```python
from build123d import *

# Parameters (mm, degrees)
SKETCH1_W           = 220
SKETCH1_H           = 145
BOSS_EXTRUDE1_DEPTH = 3
SKETCH2_W           = 220
SKETCH2_H           = 145
BOSS_EXTRUDE2_DEPTH = 12


with BuildPart() as part:
    # Sketch1 → Boss-Extrude1 (new body)
    with BuildSketch(Plane(origin=(0, 0, 0), x_dir=(1, 0, 0), z_dir=(0, 1, 0))):
        with Locations((110, 72.5)):
            Rectangle(SKETCH1_W, SKETCH1_H)
    extrude(amount=BOSS_EXTRUDE1_DEPTH)

    # Sketch2 → Boss-Extrude2 (add)
    with BuildSketch(Plane(origin=(0, 3, 0), x_dir=(1, 0, 0), z_dir=(0, 1, 0))):
        with Locations((110, 72.5)):
            Rectangle(SKETCH2_W, SKETCH2_H)
        with BuildLine():
            Line((3, 123.3), (3, 21.7))
            ThreePointArc((3, 21.7), (9.01040764, 19.21040764), (11.5, 13.2))
            Line((11.5, 13.2), (11.5, 3))
            Line((11.5, 3), (208.5, 3))
            Line((208.5, 3), (208.5, 13.2))
            ThreePointArc((208.5, 13.2), (210.98959236, 19.21040764), (217, 21.7))
            Line((217, 21.7), (217, 123.3))
            ThreePointArc((217, 123.3), (210.98959236, 125.78959236), (208.5, 131.8))
            Line((208.5, 131.8), (208.5, 142))
            Line((208.5, 142), (11.5, 142))
            Line((11.5, 142), (11.5, 131.8))
            ThreePointArc((11.5, 131.8), (9.01040764, 125.78959236), (3, 123.3))
        make_face(mode=Mode.SUBTRACT)
    extrude(amount=BOSS_EXTRUDE2_DEPTH)


solid = part.part
```
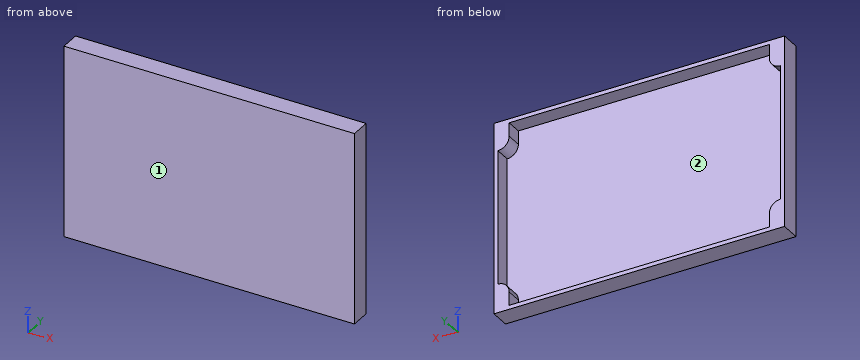
Check sheet for the modelled part. Datum: model origin and axes. Units: mm. Face numbers are marked on the shaded views. Give positions to 0.01 mm unless a question says otherwise; leave off trailing zeros. Write each loop counter-clockwise with the first axis right and the second up, starting at its lowest first coordinate (ties: lowest second). Pieces come first, ordered by that corner, then holes. Notation, with made-up numbers: (33.5, -15.5) - (91.5, -15.5) arc R29 ccw to (91.5, 9.5) - close; hole circle Ø2 at (67.5, 0). An arc over 180 degrees is marked (long way). Answer as a JSON object with one key per item and string values. Group by question number.
1) Sectioned sample at A-A (y = 6). Record the cut outline in (x, z).
2) Sectioned sample at B-B (z = -39). Record the cut outline in (x, y).
3) Release check for a two-part mould opening along Z. For the marked faces 1 and 2 record: pulls with the +Z half, pulls with the -Z half, needs draft (parallel to the pull), parting line crosses it, or undercut.
4) Depth check by flat-ended pin: P1, Ø1.5, axis at x = 47.5, z = -73.5, coming from the +Y side. Enter the tip coordinate at first touch or a pass-through.
5) Thickness scan on probe 1 along Z at (x, y) = (185.5, 5.25); probe 2 along X at (y, z) = (4, -46); probe 3 along X at (y, z) = (6.5, -136). Record the ranges inside material, lowest first. Write a range as from..to.
6) Sectioned sample at C-C (x = 169). Record the cut outline in (y, z), then the cut area to 3 significant figures.
Geometry results:
{
 "1": {"outline": "(0, -145) - (220, -145) - (220, 0) - (0, 0) - close; hole (3, -123.3) arc R8.5 cw to (11.5, -131.8) - (11.5, -142) - (208.5, -142) - (208.5, -131.8) arc R8.5 cw to (217, -123.3) - (217, -21.7) arc R8.5 cw to (208.5, -13.2) - (208.5, -3) - (11.5, -3) - (11.5, -13.2) arc R8.5 cw to (3, -21.7) - close"},
 "2": {"outline": "(0, 0) - (220, 0) - (220, 15) - (217, 15) - (217, 3) - (3, 3) - (3, 15) - (0, 15) - close"},
 "3": {"face 1": "needs draft", "face 2": "undercut"},
 "4": {"P1": "stops at y = 3"},
 "5": {"probe 1": "z = -145..-142, -3..0", "probe 2": "x = 0..3, 217..220", "probe 3": "x = 0..11.5, 208.5..220"},
 "6": {"outline": "(0, -145) - (15, -145) - (15, -142) - (3, -142) - (3, -3) - (15, -3) - (15, 0) - (0, 0) - close", "area": "507 mm^2"}
}
